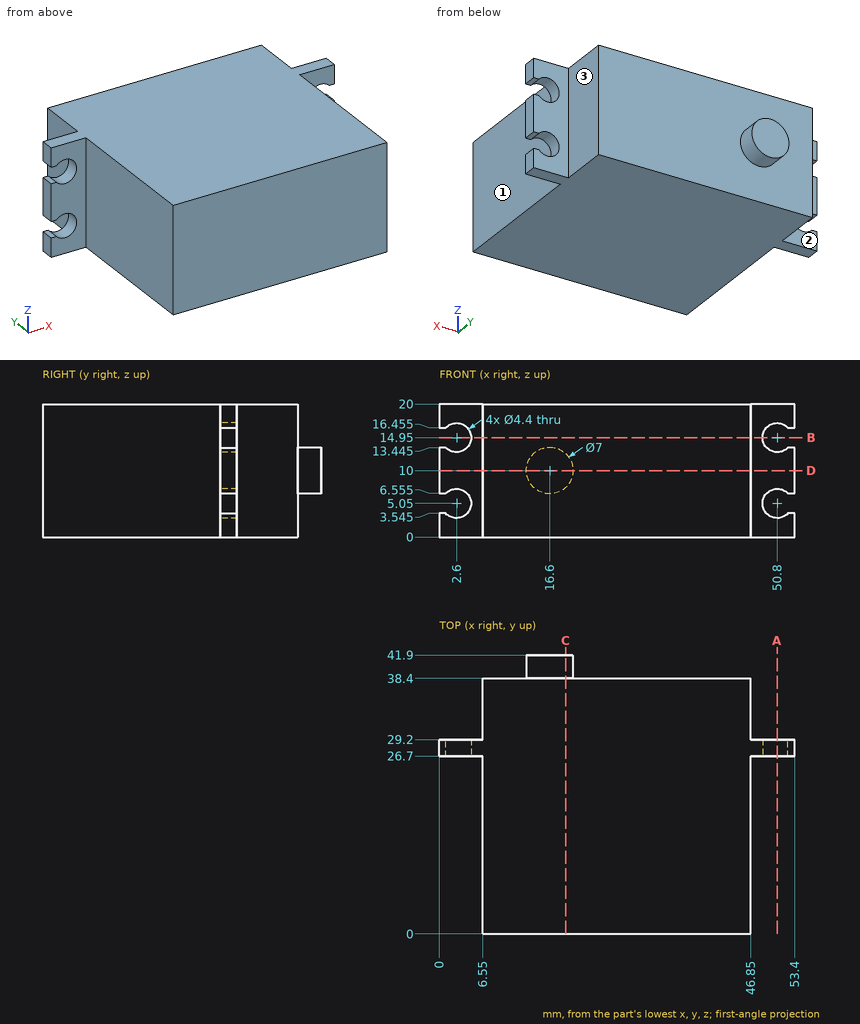
Check sheet for the drawn part. Datum: minimum x, y, z corner. Units: mm. A direction names the side the tool comes from. Round coordinates to 2 decimals unless told otherwise and drop trailing zeros. Order: outer loops, then holes, each group sorted by start corner. A loop starts at its lowest first (then second) coordinate and runs counter-clockwise, first axis right, second up. Notation, with made-up numbers: (39.25, -32) - (55.25, -32) arc R36 cw to (55.25, 2) - close; hole circle Ø4 at (28.5, 49). An arc over 180 degrees is marked (long way). Use a Markdown table: item, result. Add a question column.
(1) Sectioned sample at D-D, the plane z = 10. Enter the section's corners in (x, y).
(2) Sectioned sample at A-A, the plane x = 50.8. Enter the section's corners in (y, z).
(3) Sectioned sample at C-C, the plane x = 19. Enter the section's corners in (y, z), and give its area (3 significant figures).
(4) Depth check by flat-ended pin: pin 1 (5 mm diameter, centred on x = 2, z = 14.5, fed in from -Y); pin 2 (4.5 mm diameter, centred on y = 36, z = 15, fed in from -X); pin 3 (4 mm diameter, centred on x = 2.6, z = 5.05, fed in from +Y); pin 4 (10 mm diameter, centred on y = 8.5, z = 12.5, fed in from +X). Enter the tip coordinate at first touch or a pass-through.
(5) Material ranges on line 1 along Z through (x, y) = (2.6, 28.3); line 2 along Y through (x, z) = (33.5, 1); line 3 along X through (y, z) = (5.5, 8), recorded low to high. Write a range as [from, to].
(6) Sectioned sample at B-B, the plane z = 14.95. Enter the section's corners in (x, y).
(7) Tool access check on the marked faces 1, 2 and 3. Record the directions out of +Z, -Z, +X, -X, +Y, -Y that give a thin tool (end or side, any length) a straight path to the whole face; none if there is none.
Answers below:
| question | item | result |
|---|---|---|
| 1 | outline | (0, 26.7) - (6.55, 26.7) - (6.55, 0) - (46.85, 0) - (46.85, 26.7) - (53.4, 26.7) - (53.4, 29.2) - (46.85, 29.2) - (46.85, 38.4) - (20.1, 38.4) - (20.1, 41.9) - (13.1, 41.9) - (13.1, 38.4) - (6.55, 38.4) - (6.55, 29.2) - (0, 29.2) - close |
| 2 | outline | (26.7, 0) - (29.2, 0) - (29.2, 2.85) - (26.7, 2.85) - close; (26.7, 7.25) - (29.2, 7.25) - (29.2, 12.75) - (26.7, 12.75) - close; (26.7, 17.15) - (29.2, 17.15) - (29.2, 20) - (26.7, 20) - close |
| 3 | outline | (0, 0) - (38.4, 0) - (38.4, 7.45) - (41.9, 7.45) - (41.9, 12.55) - (38.4, 12.55) - (38.4, 20) - (0, 20) - close |
| 3 | area | 786 mm² |
| 4 | pin 1 | y = 26.7 |
| 4 | pin 2 | x = 6.55 |
| 4 | pin 3 | through |
| 4 | pin 4 | x = 46.85 |
| 5 | line 1 | [0, 2.85], [7.25, 12.75], [17.15, 20] |
| 5 | line 2 | [0, 38.4] |
| 5 | line 3 | [6.55, 46.85] |
| 6 | outline | (4.8, 26.7) - (6.55, 26.7) - (6.55, 0) - (46.85, 0) - (46.85, 26.7) - (48.6, 26.7) - (48.6, 29.2) - (46.85, 29.2) - (46.85, 38.4) - (6.55, 38.4) - (6.55, 29.2) - (4.8, 29.2) - close |
| 7 | face 1 | +Z, -Z, +X, -Y |
| 7 | face 2 | +Z, -Z, -X, +Y |
| 7 | face 3 | +Z, -Z, +X, +Y |
